```python
from build123d import *

# Parameters (mm, degrees)
BASE_FLANGE1_DEPTH = 25.4
SKETCH6_R          = 6.5024
SKETCH6_R_2        = 1.95453
CUT_EXTRUDE1_DEPTH = 69.391593051
SKETCH7_R          = 3.175
CUT_EXTRUDE2_DEPTH = 67.675


# Sheet-metal steps are written as plain solids
with BuildPart() as part:
    # Sketch1 → Base-Flange1 (new, symmetric)
    with BuildSketch(Plane(origin=(0, 0, 0), x_dir=(0, 0, -1), z_dir=(1, 0, 0))):
        with BuildLine():
            Line((0, 38.1), (0, 3.9116))
            ThreePointArc((0, 3.9116), (1.145681115, 1.145681115), (3.9116, 0))
            Line((3.9116, 0), (50.8, 0))
            Line((50.8, 0), (50.8, 3.175))
            Line((50.8, 3.175), (3.9116, 3.175))
            ThreePointArc((3.9116, 3.175), (3.390745145, 3.390745145), (3.175, 3.9116))
            Line((3.175, 3.9116), (3.175, 38.1))
            Line((3.175, 38.1), (0, 38.1))
        make_face()
    extrude(amount=BASE_FLANGE1_DEPTH, both=True)

    # Sketch6 → Cut-Extrude1 (cut, through all)
    with BuildSketch(Plane.XY):
        with Locations((0, 19.05)):
            Circle(SKETCH6_R)
        with Locations((-6.985, 26.035)):
            Circle(SKETCH6_R_2)
        with Locations((6.985, 26.035)):
            Circle(SKETCH6_R_2)
        with Locations((6.985, 12.065)):
            Circle(SKETCH6_R_2)
        with Locations((-6.985, 12.065)):
            Circle(SKETCH6_R_2)
    extrude(amount=-CUT_EXTRUDE1_DEPTH, mode=Mode.SUBTRACT)

    # Sketch7 → Cut-Extrude2 (cut, through all)
    with BuildSketch(Plane(origin=(0, 3.175, 0), x_dir=(1, 0, 0), z_dir=(0, 1, 0))):
        with Locations(Location((-19.05, 44.45, 0), (0, 0, 270))):
            Circle(SKETCH7_R)
        with Locations(Location((-19.05, 9.525, 0), (0, 0, 270))):
            Circle(SKETCH7_R)
        with Locations(Location((19.05, 44.45, 0), (0, 0, 270))):
            Circle(SKETCH7_R)
        with Locations(Location((19.05, 9.525, 0), (0, 0, 270))):
            Circle(SKETCH7_R)
    extrude(amount=-CUT_EXTRUDE2_DEPTH, mode=Mode.SUBTRACT)


solid = part.part
```
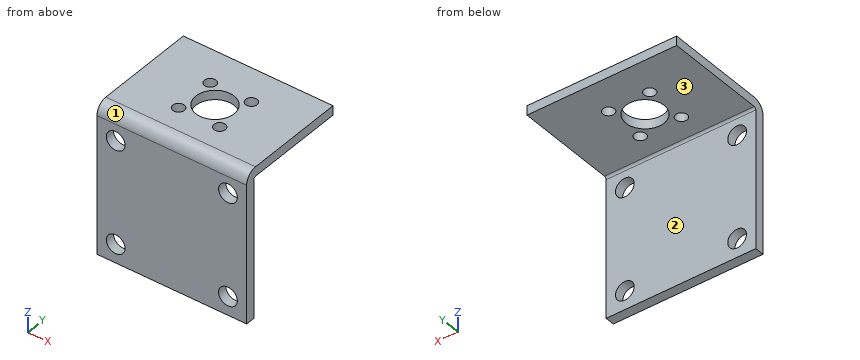
Part model, mm, in its own coordinate system. Face numbers are marked on the shaded views. Coordinates: 2 decimals unless noted, no trailing zeros. Order: outer loops, then holes, each group sorted by start corner. A loop starts at its lowest first (then second) coordinate and runs counter-clockwise, first axis right, second up. Notation, with made-up numbers: (-36, 18.5) - (15, 18.5) arc R21 ccw to (15, 50.5) - close; hole circle Ø1 at (-28, 26). An arc over 180 degrees is marked (long way). Return JSON: item names as keys, results as strings. Group by question number.
Item 1: Pull direction Z, two halves, no side cores. Call the marked faces 1, 2 and 3: pulls with the +Z half, pulls with the -Z half, needs draft (parallel to the pull), parting line crosses it, or undercut.
Item 2: Cut at A-A (z = -44.45). List the corners of the cut face in (x, y) (3 decimals), plus the area to 3 significant figures.
Item 3: Cut at C-C (y = 19.05). List the corners of the cut face in (x, z) (3 decimals).
Item 4: Cut at B-B (x = 19.05). List the corners of the cut face in (y, z) (3 decimals), plus the area to 3 significant figures.
Item 5: Pin check, flat tips, straight feed: pin 1 (4.5 mm diameter, centred on x = -6.985, y = 26.035, fed in from -Z) (3 decimals); pin 2 (6 mm diameter, centred on x = -17.5, z = -42.5, fed in from +Y) (3 decimals). Stop position of each tip, or through.
Item 6: Cut at D-D (x = 0). List the corners of the cut face in (y, z) (3 decimals).
Item 7: Drill centre lines: probe 1 along X at (y, z) = (0.9, -44.45) (3 decimals); probe 2 along Z at (x, y) = (10, 14) (3 decimals); probe 3 along Y at (x, z) = (3.5, -22.5) (3 decimals). Where is each one in solid material? Low to high. Write a range as from..to.
Check values:
{
 "1": {"face 1": "pulls with the +Z half", "face 2": "needs draft", "face 3": "pulls with the -Z half"},
 "2": {"outline": "(-25.4, 0) - (-22.225, 0) - (-22.225, 3.175) - (-25.4, 3.175) - close; (-15.875, 0) - (15.875, 0) - (15.875, 3.175) - (-15.875, 3.175) - close; (22.225, 0) - (25.4, 0) - (25.4, 3.175) - (22.225, 3.175) - close", "area": "121 mm2"},
 "3": {"outline": "(-25.4, -3.175) - (-6.502, -3.175) - (-6.502, 0) - (-25.4, 0) - close; (6.502, -3.175) - (25.4, -3.175) - (25.4, 0) - (6.502, 0) - close"},
 "4": {"outline": "(0, -50.8) - (3.175, -50.8) - (3.175, -47.625) - (0, -47.625) - close; (0, -41.275) - (3.175, -41.275) - (3.175, -12.7) - (0, -12.7) - close; (0, -6.35) - (3.175, -6.35) - (3.175, -3.912) arc R0.737 cw to (3.912, -3.175) - (38.1, -3.175) - (38.1, 0) - (3.912, 0) arc R3.912 ccw to (0, -3.912) - close", "area": "229 mm2"},
 "5": {"pin 1": "stops at z = -3.175", "pin 2": "stops at y = 3.175"},
 "6": {"outline": "(0, -50.8) - (3.175, -50.8) - (3.175, -3.912) arc R0.737 cw to (3.912, -3.175) - (12.548, -3.175) - (12.548, 0) - (3.912, 0) arc R3.912 ccw to (0, -3.912) - close; (25.552, -3.175) - (38.1, -3.175) - (38.1, 0) - (25.552, 0) - close"},
 "7": {"probe 1": "x = -25.4..-22.225, -15.875..15.875, 22.225..25.4", "probe 2": "z = -3.175..0", "probe 3": "y = 0..3.175"}
}
